from build123d import *

# Parameters (mm, degrees)
SKETCH_W      = 50.5
SKETCH_H      = 49
SKETCH_R      = 11
SKETCH_R_2    = 2.55
PAD_DEPTH     = 5
SKETCH001_W   = 25
SKETCH001_H   = 15
PAD001_DEPTH  = 10
SKETCH002_R   = 2.55
POCKET_DEPTH  = 12.5
FILLET_R      = 4.99
FILLET001_R   = 2
CHAMFER_ANGLE = 50
CHAMFER_SIZE  = 2


with BuildPart() as part:
    # Sketch → Pad (new body)
    with BuildSketch(Plane.XY):
        with Locations((0, -0.7)):
            Rectangle(SKETCH_W, SKETCH_H)
        Circle(SKETCH_R, mode=Mode.SUBTRACT)
        with Locations((-15.875, 12.7)):
            Circle(SKETCH_R_2, mode=Mode.SUBTRACT)
        with Locations((15.875, 12.7)):
            Circle(SKETCH_R_2, mode=Mode.SUBTRACT)
        with Locations((15.875, -12.7)):
            Circle(SKETCH_R_2, mode=Mode.SUBTRACT)
        with Locations((-15.875, -12.7)):
            Circle(SKETCH_R_2, mode=Mode.SUBTRACT)
    extrude(amount=PAD_DEPTH)

    # Sketch001 → Pad001 (join)
    with BuildSketch(Plane.XY):
        with Locations((0, -32.7)):
            Rectangle(SKETCH001_W, SKETCH001_H)
    extrude(amount=PAD001_DEPTH)

    # Sketch002 → Pocket (cut, symmetric)
    with BuildSketch(Plane.YZ):
        with Locations((-33, 5)):
            Circle(SKETCH002_R)
    extrude(amount=POCKET_DEPTH, both=True, mode=Mode.SUBTRACT)

    # Fillet
    fillet_edges = [part.edges().sort_by_distance(p)[0] for p in [
        (0, -25.2, 10),
        (0, -40.2, 10),
        (0, -40.2, 0),
    ]]
    fillet(fillet_edges, radius=FILLET_R)

    # Fillet001
    fillet001_edges = [part.edges().sort_by_distance(p)[0] for p in [
        (25.25, 23.8, 2.5),
        (25.25, -25.2, 2.5),
        (-25.25, 23.8, 2.5),
        (-25.25, -25.2, 2.5),
    ]]
    fillet(fillet001_edges, radius=FILLET001_R)

    # Chamfer
    chamfer_edges = [part.edges().sort_by_distance(p)[0] for p in [
        (-18.425, 12.7, 0),
        (-18.425, -12.7, 0),
        (13.325, -12.7, 0),
        (13.325, 12.7, 0),
    ]]
    chamfer_side = part.faces().sort_by_distance((0, 23.096349, 0))[0]
    chamfer(chamfer_edges, length=CHAMFER_SIZE, angle=CHAMFER_ANGLE, reference=chamfer_side)


solid = part.part
Verification items for the finished model (mm, model axes). A direction names the side the tool comes from. Give positions to 0.01 mm unless a question says otherwise; leave off trailing zeros. Write each loop counter-clockwise with the first axis right and the second up, starting at its lowest first coordinate (ties: lowest second). Pieces come first, ordered by that corner, then holes.
(1) Mould release check, pull along Y, two halves, no side actions. Record for faces 1 (the face through (25.25, -1, 2)), 2 (the face through (-2.38, -10.74, 2.46)), 3 (the face through (24.65, 23.23, 2.54)): +Y half, -Y half, draft (parallel to the pull), parting line (faces both ways), or undercut.
(2) Gauge pin test, flat ends, axial feed: pin 1 (1 mm diameter, centred on x = 11.5, y = -26, fed in from +Z); pin 2 (2 mm diameter, centred on y = -26.5, z = 5.5, fed in from -X); pin 3 (2.5 mm diameter, centred on x = -19.5, z = 2.5, fed in from -Y); pin 4 (3 mm diameter, centred on x = -15.875, y = -12.7, fed in from +Z). Record the tip position at first contact, or that the pin passes through.
(3) Cross-section at B-B (y = -33). Enter the section's corners in (x, z), plus the area to 4 significant figures.
(4) Material ranges on line 1 (Y direction, x = 0, z = 3.5); line 2 (Y direction, x = -16, z = 4); line 3 (X direction, y = 13, z = 4.5), recorded low to high.
(5) Cross-section at D-D (y = 0). Enter the section's corners in (x, z).
(6) Cross-section at A-A (x = 0). State how many separate pieces and enclosed holes the cut face has, plus the area to 3 significant figures.
(7) Access from +Z, -Z, +X, -X, +Y, -Y to the whole of each face (thin tool, end or side, straight path). Record for faces 4 (the face through (-14.452, -10.468, 2.268)), 5 (the face through (-0.4, -11.2, 5)), 6 (the face through (-12.5, -31, 3)).
Worked out:
1. face 1: draft
1. face 2: undercut
1. face 3: +Y half
2. pin 1: stops at z = 8.37
2. pin 2: stops at x = -12.5
2. pin 3: stops at y = -25.2
2. pin 4: passes through
3. outline: (-12.5, 0) - (12.5, 0) - (12.5, 2.45) - (-12.5, 2.45) - close; (-12.5, 7.55) - (12.5, 7.55) - (12.5, 10) - (-12.5, 10) - close
3. area: 122.5 mm2
4. line 1: y = -39.97 to -35.06, -30.94 to -11, 11 to 23.8
4. line 2: y = -25.2 to -15.25, -10.15 to 10.15, 15.25 to 23.8
4. line 3: x = -25.25 to -18.41, -13.34 to 13.34, 18.41 to 25.25
5. outline: (-25.25, 0) - (-11, 0) - (-11, 5) - (-25.25, 5) - close; (11, 0) - (25.25, 0) - (25.25, 5) - (11, 5) - close
6. separate pieces: 2
6. enclosed holes: 1
6. area: 249 mm2
7. face 4: -Z
7. face 5: +Z, +X, -X, +Y
7. face 6: +Z, -Z, -X, -Y
